Read the model definition and answer for the solid it produces. Units are mm, in the model's axes. A direction names the side the tool comes from. Give positions to 0.01 mm unless a question says otherwise; leave off trailing zeros. Write each loop counter-clockwise with the first axis right and the second up, starting at its lowest first coordinate (ties: lowest second). Pieces come first, ordered by that corner, then holes. Notation, with made-up numbers: (27, -31.75) -> (69, -31.75) arc R13 cw to (69, -22.75) -> close; hole circle Ø8 at (42, 71). An arc over 180 degrees is marked (long way). Put each result on its own line as item: value. Start each with the question number.
from build123d import *

# Parameters (mm, degrees)
SKETCH1_W           = 180.975
SKETCH1_H           = 38.1
SKETCH1_R           = 6.35
SKETCH1_R_2         = 1.7272
SKETCH1_R_3         = 4.2164
BOSS_EXTRUDE1_DEPTH = 19.05
SKETCH2_R           = 5.969
CUT_EXTRUDE2_DEPTH  = 8.255
SKETCH3_R           = 17.4625
CUT_EXTRUDE3_DEPTH  = 11.1125


with BuildPart() as part:
    # Sketch1 → Boss-Extrude1 (new body)
    with BuildSketch(Plane(origin=(0, 0, 0), x_dir=(0, 0, -1), z_dir=(1, 0, 0))):
        Rectangle(SKETCH1_W, SKETCH1_H)
        with Locations(Location((0, 0, 0), (0, 0, 180))):
            Circle(SKETCH1_R, mode=Mode.SUBTRACT)
        with Locations(Location((-25.4, 0, 0), (0, 0, 180))):
            Circle(SKETCH1_R_2, mode=Mode.SUBTRACT)
        with Locations(Location((-84.1375, 10.16, 0), (0, 0, 180))):
            Circle(SKETCH1_R_3, mode=Mode.SUBTRACT)
        with Locations(Location((-84.1375, -10.16, 0), (0, 0, 180))):
            Circle(SKETCH1_R_3, mode=Mode.SUBTRACT)
        with Locations(Location((25.4, 0, 0), (0, 0, 180))):
            Circle(SKETCH1_R_2, mode=Mode.SUBTRACT)
        with Locations(Location((84.1375, -10.16, 0), (0, 0, 180))):
            Circle(SKETCH1_R_3, mode=Mode.SUBTRACT)
        with Locations(Location((84.1375, 10.16, 0), (0, 0, 180))):
            Circle(SKETCH1_R_3, mode=Mode.SUBTRACT)
    extrude(amount=BOSS_EXTRUDE1_DEPTH)

    # Sketch2 → Cut-Extrude2 (cut)
    with BuildSketch(Plane(origin=(19.05, 0, 0), x_dir=(0, 0, -1), z_dir=(1, 0, 0))):
        with Locations((-84.1375, 10.16)):
            Circle(SKETCH2_R)
        with Locations(Location((-84.1375, -10.16, 0), (0, 0, 180))):
            Circle(SKETCH2_R)
        with Locations((84.1375, -10.16)):
            Circle(SKETCH2_R)
        with Locations(Location((84.1375, 10.16, 0), (0, 0, 180))):
            Circle(SKETCH2_R)
    extrude(amount=-CUT_EXTRUDE2_DEPTH, mode=Mode.SUBTRACT)

    # Sketch3 → Cut-Extrude3 (cut)
    with BuildSketch(Plane(origin=(19.05, 0, 0), x_dir=(0, 0, -1), z_dir=(1, 0, 0))):
        Circle(SKETCH3_R)
    extrude(amount=-CUT_EXTRUDE3_DEPTH, mode=Mode.SUBTRACT)


solid = part.part
1) A cutting plane is placed at A-A on z = -25.4. Give the vertices of the cut face in (x, y).
2) Straight lines are drawn through the part: line 1 (Z direction, x = 4, y = -10.16); line 2 (Z direction, x = 3, y = 10.5); line 3 (Y direction, x = 11, z = 25.4). For each, find the intervals that lie inside material, in ascending order. Write a range as [from, to].
3) A cutting plane is placed at D-D on z = 0. Give the vertices of the cut face in (x, y), and give its area (3 significant figures).
4) This flat-tipped pin is pushed along its axis until it touches: pin 1 Ø11 at (y, z) = (-10.16, 84.14) entering from +X (3 decimals). Where does it stop, or does it pass through?
5) For faces 1 (the face through (0, 9, 1)), 2 (the face through (15, 9.9, -90.1)), determine the directions among +Z, -Z, +X, -X, +Y, -Y from which every point of the face is accessible in a straight line to the end or side of a thin tool.
6) A cutting plane is placed at B-B on x = 15.5. State how many separate pieces and enclosed holes the cut face has, and give its area (3 significant figures).
7) For a pull along Z with two mould halves and no side action, classify faces 3 (the face through (9, 0, 90.488)), 4 (the face through (19.05, 0, -19)), 5 (the face through (9.392, 0.662, -23.805)), 6 (the face through (9, 0, -90.488)) as pulls with the +Z half, pulls with the -Z half, needs draft (parallel to the pull), parting line crosses it, or undercut.
Results found:
1. outline: (0, -19.05) -> (19.05, -19.05) -> (19.05, -1.73) -> (0, -1.73) -> close; (0, 1.73) -> (19.05, 1.73) -> (19.05, 19.05) -> (0, 19.05) -> close
2. line 1: z = [-90.49, -88.35], [-79.92, 79.92], [88.35, 90.49]
2. line 2: z = [-90.49, -88.34], [-79.93, 79.93], [88.34, 90.49]
2. line 3: y = [-19.05, -1.73], [1.73, 19.05]
3. outline: (0, -19.05) -> (19.05, -19.05) -> (19.05, -17.46) -> (7.94, -17.46) -> (7.94, -6.35) -> (0, -6.35) -> close; (0, 6.35) -> (7.94, 6.35) -> (7.94, 17.46) -> (19.05, 17.46) -> (19.05, 19.05) -> (0, 19.05) -> close
3. area: 237 mm²
4. pin 1: stops at x = 10.795
5. face 1: +Z, -Z, -X, +Y, -Y
5. face 2: +X
6. separate pieces: 1
6. enclosed holes: 7
6. area: 5,470 mm²
7. face 3: pulls with the +Z half
7. face 4: needs draft
7. face 5: undercut
7. face 6: pulls with the -Z half
